Input: part model. Units: mm. Frame: model coordinates. A direction names the side the tool comes from. Give positions to 0.01 mm unless a question says otherwise; leave off trailing zeros. Loops run counter-clockwise (first coordinate to the right, second up) from the corner with the lowest first, then second, coordinate; pieces in that order, holes last. Notation, with made-up numbers: M -39.75,76.25 L -7.75,76.25 A27 ccw -7.75,103.25 Z; hole C 8,18 d7. An arc over 180 degrees is marked long. Answer as a JSON object with one key per item and string values. Group by question number.
1) Draft query along Y for faces 4 (the cylindrical face through (-30.76, 102.463, -51.574)), 5 (the cylindrical face through (-30.76, 84.668, -39.904)), 6 (the cylindrical face through (0.975, 4.437, 133.212)). Return one class per face: +Y half, -Y half, draft (parallel to the pull), parting line (faces both ways), or undercut.
2) Section query A-A on z = -50.96. Return loops of the section in (x, y), plus the area to 3 significant figures.
3) Ray query, L1, parallel to Y at x = -32.5, z = -50.96; L2, parallel to Y at x = -29, z = -50; L3, parallel to Z at x = -33, y = 74. Return the intervals inside material, ascending.
4) Section query D-D on y = 18. Return loops of the section in (x, z), plus the area to 3 significant figures.
5) Section query C-C on x = 0. Return loops of the section in (y, z), plus the area to 3 significant figures.
6) Section query B-B on y = 86. Return loops of the section in (x, z), plus the area to 3 significant figures.
7) Access query for faces 1 (the flat face through (-31, 41, -78.9)), 2 (the flat face through (-26.323, 45, -51)), 3 (the flat face through (-31, 41, -23.02)). Directions: +Z, -Z, +X, -X, +Y, -Y. A direction counts if a zero-diameter tool reaches every point of the face in a straight line with its end or side. Return the directions, or none.
8) First-contact query: P1, Ø7, axis at x = -31.5, y = 44, coming from the +Z side; P2, Ø17, axis at y = 59, z = -37.5, coming from the +X side; P3, Ø4.5, axis at x = -29, y = 33.5, coming from the -Z side. Flat tips, straight axial feed; report the tip coordinate or a pass-through.
from build123d import *

# Parameters (mm, degrees)
BOSS_EXTRUDE1_DEPTH = 9
SKETCH2_W           = 9
SKETCH2_H           = 55.88
BOSS_EXTRUDE2_DEPTH = 65.53
SKETCH3_R           = 27.94
BOSS_EXTRUDE3_DEPTH = 9
SKETCH4_R           = 15
CUT_EXTRUDE1_DEPTH  = 19


with BuildPart() as part:
    # Sketch1 → Boss-Extrude1 (new body)
    with BuildSketch(Plane(origin=(0, 0, 0), x_dir=(1, 0, 0), z_dir=(0, 1, 0))):
        with BuildLine():
            Line((44.323, 88.9), (44.323, -88.9))
            ThreePointArc((44.323, -88.9), (0, -133.223), (-44.323, -88.9))
            Line((-44.323, -88.9), (-44.323, 88.9))
            ThreePointArc((-44.323, 88.9), (0, 133.223), (44.323, 88.9))
        make_face()
    extrude(amount=BOSS_EXTRUDE1_DEPTH)

    # Sketch2 → Boss-Extrude2 (add)
    with BuildSketch(Plane(origin=(0, 9, 0), x_dir=(1, 0, 0), z_dir=(0, 1, 0))):
        with Locations((-30.823, 50.96)):
            Rectangle(SKETCH2_W, SKETCH2_H)
    extrude(amount=BOSS_EXTRUDE2_DEPTH)

    # Sketch3 → Boss-Extrude3 (add)
    with BuildSketch(Plane(origin=(-26.323, 0, 0), x_dir=(0, 0, -1), z_dir=(1, 0, 0))):
        with Locations((50.96, 74.53)):
            Circle(SKETCH3_R)
    extrude(amount=-BOSS_EXTRUDE3_DEPTH)

    # Sketch4 → Cut-Extrude1 (cut, through all)
    with BuildSketch(Plane(origin=(-26.323, 0, 0), x_dir=(0, 0, -1), z_dir=(1, 0, 0))):
        with Locations((50.96, 74.53)):
            Circle(SKETCH4_R)
    extrude(amount=-CUT_EXTRUDE1_DEPTH, mode=Mode.SUBTRACT)


solid = part.part
Output:
{
 "1": {"face 4": "+Y half", "face 5": "undercut", "face 6": "draft"},
 "2": {"outline": "M -44.32,0 L 44.32,0 L 44.32,9 L -26.32,9 L -26.32,59.53 L -35.32,59.53 L -35.32,9 L -44.32,9 Z; M -35.32,89.53 L -26.32,89.53 L -26.32,102.47 L -35.32,102.47 Z", "area": "1,370 mm^2"},
 "3": {"L1": "y = 0 to 59.53, 89.53 to 102.47", "L2": "y = 0 to 59.56, 89.5 to 102.45", "L3": "z = -78.9 to -65.95, -35.97 to -23.02"},
 "4": {"outline": "M -35.32,-78.9 L -26.32,-78.9 L -26.32,-23.02 L -35.32,-23.02 Z", "area": "503 mm^2"},
 "5": {"outline": "M 0,-133.22 L 9,-133.22 L 9,133.22 L 0,133.22 Z", "area": "2,400 mm^2"},
 "6": {"outline": "M -35.32,-76.44 L -26.32,-76.44 L -26.32,-60.63 L -35.32,-60.63 Z; M -35.32,-41.29 L -26.32,-41.29 L -26.32,-25.48 L -35.32,-25.48 Z", "area": "285 mm^2"},
 "7": {"face 1": "-Z, +X, -X, +Y", "face 2": "+Z, -Z, +X, +Y", "face 3": "+Z, +X, -X, +Y"},
 "8": {"P1": "stops at z = -23.02", "P2": "stops at x = -26.32", "P3": "stops at z = -78.9"}
}
